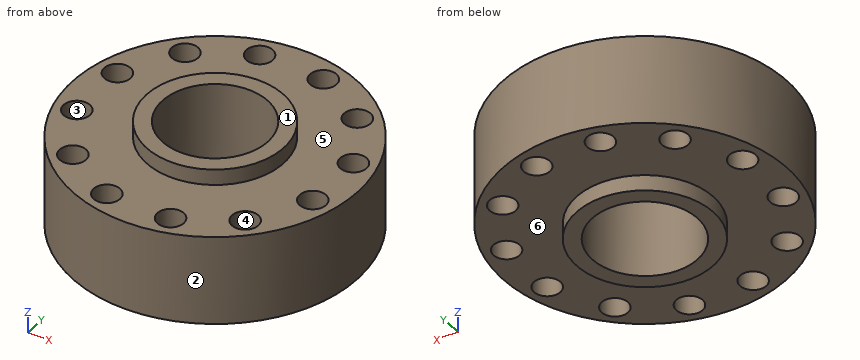
```python
from build123d import *

# Parameters (mm, degrees)
SKETCH_3_R               = 27
EXTRUDE_1_DEPTH          = 8.5
SKETCH_5_R               = 13
CUT_EXTRUDE_2_DEPTH      = 42.797129088
SKETCH_8_R               = 13
SKETCH_8_R_2             = 10
EXTRUDE_2_DEPTH          = 11.5
CUT_EXTRUDE_3_REACH      = 45.105
SKETCH_9_R               = 2.5
PATTERN_CIRCULAR_2_COUNT = 6


with BuildPart() as part:
    # Sketch 3 → Extrude 1 (new, symmetric)
    with BuildSketch(Plane.XY):
        Circle(SKETCH_3_R)
    extrude(amount=EXTRUDE_1_DEPTH, both=True)

    # Sketch 5 → Cut-Extrude 2 (cut, through all)
    with BuildSketch(Plane(origin=(0, 0, -8.5), x_dir=(-1, 0, 0), z_dir=(0, 0, -1))):
        Circle(SKETCH_5_R)
    extrude(amount=-CUT_EXTRUDE_2_DEPTH, mode=Mode.SUBTRACT)

    # Sketch 8 → Extrude 2 (add, symmetric)
    with BuildSketch(Plane.XY):
        with Locations(Location((0, 0, 0), (0, 0, 180))):
            Circle(SKETCH_8_R)
        Circle(SKETCH_8_R_2, mode=Mode.SUBTRACT)
    extrude(amount=EXTRUDE_2_DEPTH, both=True)

    # Sketch 9 → Cut-Extrude 3 (cut, up to next)
    with BuildSketch(Plane(origin=(0, 0, -8.5), x_dir=(-1, 0, 0), z_dir=(0, 0, -1)), mode=Mode.PRIVATE) as cut_extrude_3_sk1:
        with Locations((-6, 22.203603311)):
            Circle(SKETCH_9_R)
    cut_extrude_3_tool1 = extrude(cut_extrude_3_sk1.sketch, amount=-CUT_EXTRUDE_3_REACH, mode=Mode.PRIVATE) & part.part
    # Sketch 9 → Cut-Extrude 3 (cut, up to next)
    with BuildSketch(Plane(origin=(0, 0, -8.5), x_dir=(-1, 0, 0), z_dir=(0, 0, -1)), mode=Mode.PRIVATE) as cut_extrude_3_sk2:
        with Locations((6, 22.203603311)):
            Circle(SKETCH_9_R)
    cut_extrude_3_tool2 = extrude(cut_extrude_3_sk2.sketch, amount=-CUT_EXTRUDE_3_REACH, mode=Mode.PRIVATE) & part.part
    cut_extrude_3_1 = cut_extrude_3_tool1.solids().sort_by_distance((6, 22.203603, -8.5))[0]
    add(cut_extrude_3_1, mode=Mode.SUBTRACT)
    cut_extrude_3_2 = cut_extrude_3_tool2.solids().sort_by_distance((-6, 22.203603, -8.5))[0]
    add(cut_extrude_3_2, mode=Mode.SUBTRACT)
    cut_extrude_3 = cut_extrude_3_1 + cut_extrude_3_2  # Cut-Extrude 3 as one shape, for the pattern or mirror that repeats it

    # Pattern Circular 2: Cut-Extrude 3 ×6 about axis
    pattern_circular_2_axis = Axis((0, 0, 0), (0, 0, 1))
    for i in range(1, PATTERN_CIRCULAR_2_COUNT):
        add(cut_extrude_3.rotate(pattern_circular_2_axis, i * 360 / PATTERN_CIRCULAR_2_COUNT), mode=Mode.SUBTRACT)


solid = part.part
```
Model file for the job. Use its own axes, mm. Face numbers are marked on the shaded views. A direction names the side the tool comes from. Coordinates: 2 decimals unless noted, no trailing zeros. Write each loop counter-clockwise with the first axis right and the second up, starting at its lowest first coordinate (ties: lowest second). Pieces come first, ordered by that corner, then holes. Notation, with made-up numbers: (69, 60.25) - (75, 60.25) arc R5 cw to (75, 67.25) - close; hole circle Ø6 at (-6.75, 58). An arc over 180 degrees is marked (long way). Use a Markdown table: item, result. Add a question column.
Item 1: Band-saw the part on B-B, the plane x = -4.5. Write the cut outline in (y, z), and give its area (3 significant figures).
Item 2: Band-saw the part on D-D, the plane y = -6.5. Write the cut outline in (x, z), and give its area (3 significant figures).
Item 3: 3-axis set-ups, long thin cutter, end or side, ignore diameter. For the marked faces 4, 5 and 6: which of +Z, -Z, +X, -X, +Y, -Y reach the whole face in a straight line?
Item 4: Band-saw the part on A-A, the plane y = 0. Write the cut outline in (x, z), and give its area (3 significant figures).
Item 5: Band-saw the part on C-C, the plane x = 1. Write the cut outline in (y, z).
Item 6: Drop flat-ended pins along their axis: pin 1 (5 mm diameter, centred on x = 9, z = 2.5, fed in from -Y); pin 2 (1.5 mm diameter, centred on x = -12.5, z = 8, fed in from -Y); pin 3 (1 mm diameter, centred on y = 6, z = 4.5, fed in from -X). Give the stop position or say it passes through.
Item 7: Two-plate mould, pull along X, no slides. Class the marked faces 1, 2 and 3: pulls with the +X half, pulls with the -X half, needs draft (parallel to the pull), parting line crosses it, or undercut.
Item 8: Drill centre lines: line 1 along Y through (x, z) = (-6, -1.5); line 2 along X through (y, z) = (4, -7.75); line 3 along X through (y, z) = (-5, -4.75). Where is each one in solid material? Low to high.
A:
| question | item | result |
|---|---|---|
| 1 | outline | (-26.62, -8.5) - (-24.2, -8.5) - (-24.2, 8.5) - (-26.62, 8.5) - close; (-20.2, -8.5) - (-12.2, -8.5) - (-12.2, -11.5) - (-8.93, -11.5) - (-8.93, 11.5) - (-12.2, 11.5) - (-12.2, 8.5) - (-20.2, 8.5) - close; (8.93, -11.5) - (12.2, -11.5) - (12.2, -8.5) - (20.2, -8.5) - (20.2, 8.5) - (12.2, 8.5) - (12.2, 11.5) - (8.93, 11.5) - close; (24.2, -8.5) - (26.62, -8.5) - (26.62, 8.5) - (24.2, 8.5) - close |
| 1 | area | 505 mm² |
| 2 | outline | (-26.21, -8.5) - (-24.66, -8.5) - (-24.66, 8.5) - (-26.21, 8.5) - close; (-19.8, -8.5) - (-11.26, -8.5) - (-11.26, -11.5) - (-7.6, -11.5) - (-7.6, 11.5) - (-11.26, 11.5) - (-11.26, 8.5) - (-19.8, 8.5) - close; (7.6, -11.5) - (11.26, -11.5) - (11.26, -8.5) - (19.8, -8.5) - (19.8, 8.5) - (11.26, 8.5) - (11.26, 11.5) - (7.6, 11.5) - close; (24.66, -8.5) - (26.21, -8.5) - (26.21, 8.5) - (24.66, 8.5) - close |
| 2 | area | 511 mm² |
| 3 | face 4 | +Z, -Z |
| 3 | face 5 | +Z |
| 3 | face 6 | -Z |
| 4 | outline | (-27, -8.5) - (-13, -8.5) - (-13, -11.5) - (-10, -11.5) - (-10, 11.5) - (-13, 11.5) - (-13, 8.5) - (-27, 8.5) - close; (10, -11.5) - (13, -11.5) - (13, -8.5) - (27, -8.5) - (27, 8.5) - (13, 8.5) - (13, 11.5) - (10, 11.5) - close |
| 4 | area | 614 mm² |
| 5 | outline | (-26.98, -8.5) - (-12.96, -8.5) - (-12.96, -11.5) - (-9.95, -11.5) - (-9.95, 11.5) - (-12.96, 11.5) - (-12.96, 8.5) - (-26.98, 8.5) - close; (9.95, -11.5) - (12.96, -11.5) - (12.96, -8.5) - (26.98, -8.5) - (26.98, 8.5) - (12.96, 8.5) - (12.96, 11.5) - (9.95, 11.5) - close |
| 6 | pin 1 | stops at y = -26.21 |
| 6 | pin 2 | stops at y = -24.31 |
| 6 | pin 3 | stops at x = -26.43 |
| 7 | face 1 | needs draft |
| 7 | face 2 | parting line crosses it |
| 7 | face 3 | undercut |
| 8 | line 1 | y = -26.32 to -24.7, -19.7 to -8, 8 to 19.7, 24.7 to 26.32 |
| 8 | line 2 | x = -26.7 to -23.85, -20.61 to -9.17, 9.17 to 20.61, 23.85 to 26.7 |
| 8 | line 3 | x = -26.53 to -24.56, -19.9 to -8.66, 8.66 to 19.9, 24.56 to 26.53 |
